Here's how the part is built. I have some questions about the finished solid (model axes, mm). Face numbers are marked on the shaded views. Coordinates: 2 decimals unless noted, no trailing zeros. Write each loop counter-clockwise with the first axis right and the second up, starting at its lowest first coordinate (ties: lowest second). Pieces come first, ordered by that corner, then holes.
(1) Imagine slicing it at D-D, the plane y = 60.5. List the corners of the cut face in (x, z) for me.
(2) For pin 1 Ø3 at (y, z) = (51.5, 7) entering from -X; pin 2 Ø1.5 at (y, z) = (49.5, 1.5) entering from -X; pin 3 Ø4 at (y, z) = (48, 4) entering from +X, each with a flat end and sliding along its axis, tell me the tip position at first contact or that it passes through.
(3) Thinking about a two-plate mould opening in Y: for the marked faces 1, 2, 3 and 4, which applies, released by +Y, released by -Y, zero draft, split by the parting line, or undercut?
(4) Imagine slicing it at B-B, the plane y = 4. List the corners of the cut face in (x, z) for me.
(5) Imagine slicing it at C-C, the plane z = 6.75. State how many separate pieces and enclosed holes the cut face has, plus the area to 3 significant figures.
(6) Imagine slicing it at A-A, the plane x = 25. List the corners of the cut face in (y, z) for me.
(7) Please list where these lines run through material, in increasing order: probe 1 along Z at (x, y) = (12, 5); probe 2 along Y at (x, z) = (25.5, 2.75); probe 3 along X at (y, z) = (56.75, 5.5).
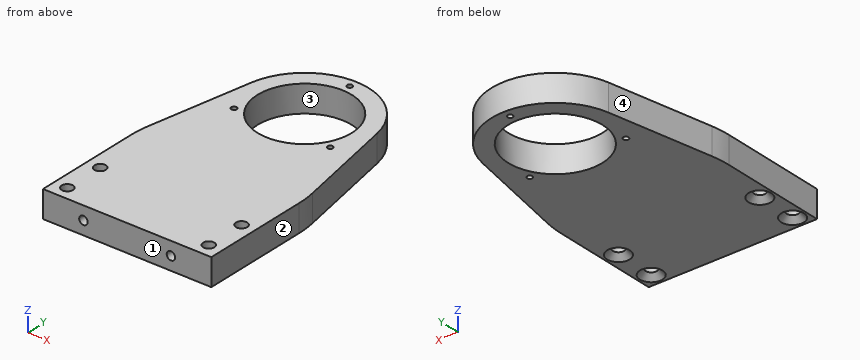
```python
from build123d import *

# Parameters (mm, degrees)
EXTRUDE_1_DEPTH              = 8
FILLET_1_R                   = 30
CUT_EXTRUDE_1_REACH          = 10
SKETCH_2_R                   = 14
HOLE_WIZARD_M3_1_D           = 3.4
HOLE_WIZARD_M3_1_DEPTH       = 8
HOLE_WIZARD_M3_1_CSINK_D     = 6.72
HOLE_WIZARD_M3_1_CSINK_ANGLE = 90
HOLE_WIZARD_M3_1_2_D         = 2.5
HOLE_WIZARD_M3_1_2_DEPTH     = 8.5
HOLE_WIZARD_M3_1_2_TIP       = 0.751075774
HOLE_WIZARD_M2_1_D           = 1.6


with BuildPart() as part:
    # 스케치1 → 보스-돌출1 (new body)
    with BuildSketch(Plane.XY):
        with BuildLine():
            Line((0, 35), (0, 0))
            Line((0, 0), (50, 0))
            Line((50, 0), (50, 35))
            Line((50, 35), (43.670126691, 68.525105576))
            ThreePointArc((43.670126691, 68.525105576), (25, 84), (6.329873309, 68.525105576))
            Line((6.329873309, 68.525105576), (0, 35))
        make_face()
    extrude(amount=EXTRUDE_1_DEPTH)

    # 필렛1
    fillet_1_edges = [part.edges().sort_by_distance(p)[0] for p in [
        (50, 35, 4),
        (0, 35, 4),
    ]]
    fillet(fillet_1_edges, radius=FILLET_1_R)

    # 스케치2 → 컷-돌출1 (cut, up to next)
    with BuildSketch(Plane(origin=(0, 0, 0), x_dir=(-1, 0, 0), z_dir=(0, 0, -1)), mode=Mode.PRIVATE) as cut_extrude_1_sk1:
        with Locations((-25, 65)):
            Circle(SKETCH_2_R)
    cut_extrude_1_tool1 = extrude(cut_extrude_1_sk1.sketch, amount=-CUT_EXTRUDE_1_REACH, mode=Mode.PRIVATE) & part.part
    add(cut_extrude_1_tool1.solids().sort_by_distance((25, 65, 0))[0], mode=Mode.SUBTRACT)

    # Hole Wizard M3 _ _ _ _ _ _ _1
    with Locations(Plane(origin=(0, 0, 0), x_dir=(-1, 0, 0), z_dir=(0, 0, -1))):
        with Locations((-4, 16), (-4, 4), (-46, 16), (-46, 4)):
            CounterSinkHole(HOLE_WIZARD_M3_1_D / 2, HOLE_WIZARD_M3_1_CSINK_D / 2, depth=HOLE_WIZARD_M3_1_DEPTH, counter_sink_angle=HOLE_WIZARD_M3_1_CSINK_ANGLE)

    # Hole Wizard M3 _ _1 2
    with Locations(Plane(origin=(0, 0, 0), x_dir=(-1, 0, 0), z_dir=(0, -1, 0))):
        with Locations((-38, -4), (-12, -4)):
            Hole(HOLE_WIZARD_M3_1_2_D / 2, depth=HOLE_WIZARD_M3_1_2_DEPTH)
            with Locations((0, 0, -(HOLE_WIZARD_M3_1_2_DEPTH + HOLE_WIZARD_M3_1_2_TIP / 2))):  # 118° drill point
                Cone(0, HOLE_WIZARD_M3_1_2_D / 2, HOLE_WIZARD_M3_1_2_TIP, mode=Mode.SUBTRACT)

    # M2 나사 구멍1 (through all)
    with Locations(Plane(origin=(0, 0, 0), x_dir=(-1, 0, 0), z_dir=(0, 0, -1))):
        with Locations((-10.710580838, 56.75), (-25, 81.5), (-39.289419162, 56.75)):
            Hole(HOLE_WIZARD_M2_1_D / 2)


solid = part.part
```
Recorded:
1. outline: (4.81, 0) - (11.74, 0) - (11.74, 8) - (4.81, 8) - close; (38.26, 0) - (45.19, 0) - (45.19, 8) - (38.26, 8) - close
2. pin 1: stops at x = 2.83
2. pin 2: stops at x = 2.6
2. pin 3: stops at x = 47.92
3. face 1: released by -Y
3. face 2: zero draft
3. face 3: undercut
3. face 4: released by +Y
4. outline: (0, 0) - (0.64, 0) - (2.3, 1.66) - (2.3, 8) - (0, 8) - close; (5.7, 1.66) - (7.36, 0) - (42.64, 0) - (44.3, 1.66) - (44.3, 8) - (5.7, 8) - close; (47.7, 1.66) - (49.36, 0) - (50, 0) - (50, 8) - (47.7, 8) - close; hole circle Ø2.5 at (12, 4); hole circle Ø2.5 at (38, 4)
5. separate pieces: 1
5. enclosed holes: 8
5. area: 2,990 mm2
6. outline: (0, 0) - (51, 0) - (51, 8) - (0, 8) - close; (79, 0) - (80.7, 0) - (80.7, 8) - (79, 8) - close; (82.3, 0) - (84, 0) - (84, 8) - (82.3, 8) - close
7. probe 1: z = 0 to 2.75, 5.25 to 8
7. probe 2: y = 0 to 51.01, 78.99 to 80.88, 82.12 to 83.99
7. probe 3: x = 4.11 to 9.91, 11.51 to 13.69, 36.31 to 38.49, 40.09 to 45.89
